Geometry: see drawing. Coordinates: mm, zero at the bounding-box minimum. A direction names the side the tool comes from. Coordinates: 2 decimals unless noted, no trailing zeros. Loops run counter-clockwise (first coordinate to the right, second up) from the corner with the lowest first, then second, coordinate; pieces in that order, holes last. Notation, with made-up numbers: (63, 68) - (91, 68) arc R29 cw to (91, 105) - close; hole circle Ø3 at (21, 56). An arc over 180 degrees is marked (long way). Use one line per item in the form item = value.
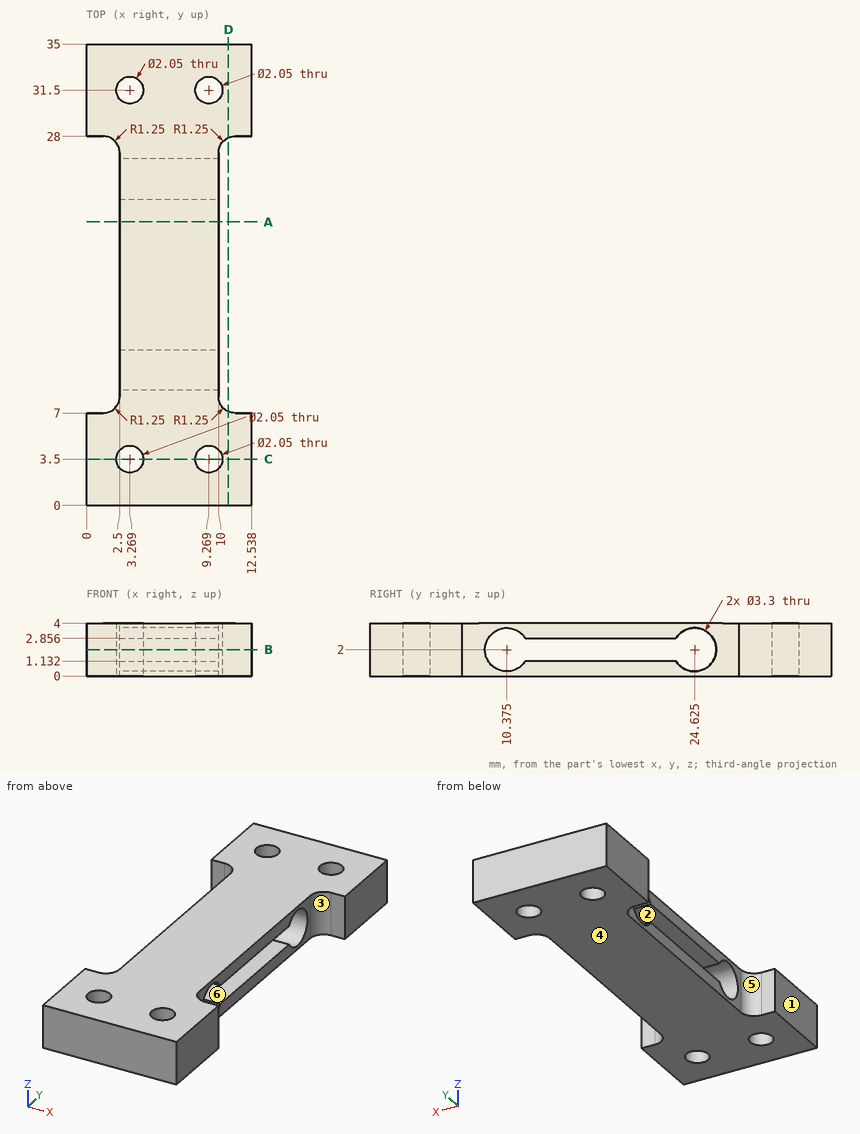
Q1. Pull-direction query (Z, two-part tool) for the marked faces 4, 5 and 6; classes: pulls with the +Z half, pulls with the -Z half, needs draft (parallel to the pull), parting line crosses it, or undercut.
Check values:
face_4 = pulls with the -Z half
face_5 = needs draft
face_6 = undercut
Q2. Cut plane C-C, the plane y = 3.5. Return loops of the section in (x, z) (1 decimal).
Check values:
outline = (0, 0) - (2.2, 0) - (2.2, 4) - (0, 4) - close; (4.3, 0) - (8.2, 0) - (8.2, 4) - (4.3, 4) - close; (10.3, 0) - (12.5, 0) - (12.5, 4) - (10.3, 4) - close
Q3. Set-up query: the marked faces 1, 2 and 3. Return all of +Z, -Z, +X, -X, +Y, -Y with unobstructed straight access to the full face (end or side cutting, diameter ignored); none if empty.
Check values:
face_1 = +Z, -Z, -X, +Y, -Y
face_2 = +X, -X
face_3 = +Z, -Z, +X
Q4. Cut plane D-D, the plane x = 10.75. Return loops of the section in (y, z) (1 decimal).
Check values:
outline = (0, 0) - (7.1, 0) - (7.1, 4) - (0, 4) - close; (27.9, 0) - (35, 0) - (35, 4) - (27.9, 4) - close
Q5. Ray query, line 1 along Y through (x, z) = (3.25, 3.8) (1 decimal); line 2 along Y through (x, z) = (12.25, 0.6); line 3 along Y through (x, z) = (6.5, 2) (1 decimal). Return the intervals inside material, ascending. Write a range as [from, to].
Check values:
line_1 = [0, 2.5], [4.5, 30.5], [32.5, 35]
line_2 = [0, 7], [28, 35]
line_3 = [0, 8.7], [26.3, 35]
Q6. First-contact query: P1, Ø2, axis at y = 20, z = 2, coming from the +X side; P2, Ø1.6, axis at x = 3.27, y = 31.5, coming from the -Z side; P3, Ø2, axis at y = 18, z = 2, coming from the -X side. Flat tips, straight axial feed; report the tip coordinate or a pass-through.
Check values:
P1 = 10
P2 = through
P3 = 2.5
Q7. Cut plane A-A, the plane y = 21.5. Return loops of the section in (x, z).
Check values:
outline = (2.5, 0) - (10, 0) - (10, 1.13) - (2.5, 1.13) - close; (2.5, 2.86) - (10, 2.86) - (10, 4) - (2.5, 4) - close
Q8. Cut plane B-B, the plane z = 2. Give the number of separate pieces and of enclosed holes in the cut face.
Check values:
separate_pieces = 2
enclosed_holes = 4
